Autodesk Inventor part; units mm, degrees
ref_plane "YZ Plane" through (0, 0, 0) normal (1, 0, 0) x (0, 1, 0)
ref_plane "XZ Plane" through (0, 0, 0) normal (0, 1, 0) x (-1, 0, 0)
ref_plane "XY Plane" through (0, 0, 0) normal (0, 0, 1) x (1, 0, 0)
sketch "Sketch1" plane through (0, 0, 0) normal (0, 0, 1) x (1, 0, 0)
  line L0 (-20, -0.7) -> (-20, 10)
  line L1 (0, 7.7) -> (0, 1.3)
  circle A0 centre (-16.5, 5) radius 1.5606
  line L2 (1.2, 6.5) -> (12.2, 6.5)
  line L3 (1.2, 2.5) -> (4.8537, 2.5)
  line L4 (1.2, 6.5) -> (1.2, 2.5)
  line L5 (0, 1.3) -> (4.8537, 1.3)
  line L6 (4.8537, 2.5) -> (4.8537, 1.3)
  line L7 (12.2, -0.7) -> (12.2, 6.5)
  line L8 (0, 7.7) -> (10, 7.7)
  line L9 (10, 7.7) -> (10, 10)
  line L10 (-20, -0.7) -> (12.2, -0.7)
  line L11 (-20, 10) -> (10, 10)
  dimension "d0" = 16.5
  dimension "d7" = 1.2
  dimension "d9" = 1.2
  dimension "d10" = 11
  dimension "d12" = 1.2
  dimension "d13" = 4
  dimension "d14" = 2
  dimension "d17" = 5
extrude "Extrusion1" add sketch "Sketch1" along normal blind 7
sketch "Sketch2" plane through (0, 0, 0) normal (0, 0, -1) x (-1, 0, 0)
  line L0 (20, 10) -> (2.1389, 10)
  line L1 (2.1389, 10) -> (2.1389, 9)
  line L2 (2.1389, 9) -> (20, 9)
  line L3 (20, 9) -> (20, 10)
  line L4 (20, 10) -> (-10, 10)
  line L5 (20, -0.7) -> (20, 10)
  point P0 (0, 0)
  dimension "d18" = 1
extrude "Extrusion2" add sketch "Sketch2" along normal blind 2
properties part number "opto mount"
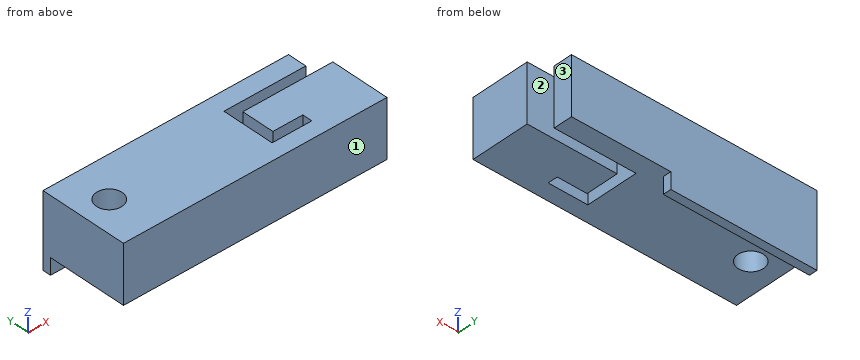
Source: CAD feature listing. Evaluate the final solid. Frame: model axes, mm. Face numbers are marked on the shaded views. Round coordinates to 2 decimals unless told otherwise and drop trailing zeros. Write each loop counter-clockwise with the first axis right and the second up, starting at its lowest first coordinate (ties: lowest second). Pieces come first, ordered by that corner, then holes. Notation, with made-up numbers: (60, -25) - (65, -25) arc R19 cw to (65, 0) - close; hole circle Ø9 at (35, 0.5). An arc over 180 degrees is marked (long way). Use CSV: the item, a comma, the result in double quotes. Start each with the question number.
(1) Cut plane C-C, the plane x = 4.5. Return loops of the section in (y, z).
(2) First-contact query: pin 1 Ø0.6 at (x, z) = (-13, -1) entering from -Y; pin 2 Ø2.5 at (y, z) = (9, 2.5) entering from +X. Flat tips, straight axial feed; report the tip coordinate or a pass-through.
(3) Cut plane A-A, the plane x = -16.5. Return loops of the section in (y, z).
(4) Cut plane D-D, the plane z = 4.5. Return loops of the section in (x, y), and give its area (3 significant figures).
(5) Mould query, pull axis Y, two halves, no side actions, for the marked faces 1, 2 and 3. Classes: pulls with the +Y half, pulls with the -Y half, needs draft (parallel to the pull), parting line crosses it, or undercut.
(6) Material intervals for probe 1 along Y at (x, z) = (3, 2.5); probe 2 along Y at (x, z) = (-16.5, 2.5); probe 3 along X at (y, z) = (4.75, 4), sorted ascending. Write a range as [from, to].
(7) Cut plane B-B, the plane y = 5. Return loops of the section in (x, z), and give its area (3 significant figures).
Geometry says:
1,outline,"(-0.7, 0) - (1.3, 0) - (1.3, 7) - (-0.7, 7) - close; (2.5, 0) - (6.5, 0) - (6.5, 7) - (2.5, 7) - close; (7.7, 0) - (10, 0) - (10, 7) - (7.7, 7) - close"
2,pin 1,"y = 9"
2,pin 2,"x = 10"
3,outline,"(-0.7, 0) - (3.44, 0) - (3.44, 7) - (-0.7, 7) - close; (6.56, 0) - (9, 0) - (9, -2) - (10, -2) - (10, 7) - (6.56, 7) - close"
4,outline,"(-20, -0.7) - (12.2, -0.7) - (12.2, 6.5) - (1.2, 6.5) - (1.2, 2.5) - (4.85, 2.5) - (4.85, 1.3) - (0, 1.3) - (0, 7.7) - (10, 7.7) - (10, 10) - (-20, 10) - close; hole circle Ø3.12 at (-16.5, 5)"
4,area,"307 mm²"
5,face 1,"pulls with the -Y half"
5,face 2,"undercut"
5,face 3,"needs draft"
6,probe 1,"[-0.7, 1.3], [2.5, 6.5], [7.7, 10]"
6,probe 2,"[-0.7, 3.44], [6.56, 10]"
6,probe 3,"[-20, -18.04], [-14.96, 0], [1.2, 12.2]"
7,outline,"(-20, 0) - (-18.06, 0) - (-18.06, 7) - (-20, 7) - close; (-14.94, 0) - (0, 0) - (0, 7) - (-14.94, 7) - close; (1.2, 0) - (12.2, 0) - (12.2, 7) - (1.2, 7) - close"
7,area,"195 mm²"
